CAD build for the part. Positions are in the model's coordinates, mm. Give positions to 0.01 mm unless a question says otherwise; leave off trailing zeros. Loops run counter-clockwise (first coordinate to the right, second up) from the corner with the lowest first, then second, coordinate; pieces in that order, holes last.
Item 1: Probe probe 1 along Z at (x, y) = (27, 2.75); probe 2 along X at (y, z) = (3.15, -56); probe 3 along Z at (x, y) = (-16, 2.35). List the from-to ranges inside material, lowest first.
Item 2: Saw through at C-C on x = -8. Give the cut face in (y, z).
Item 3: Drop flat-ended pins along their axis: P1, Ø5, axis at x = 25.54, z = -58.12, coming from the +Y side; P2, Ø2.5, axis at x = 25.54, z = 44.04, coming from the +Y side; P3, Ø2, axis at y = 1, z = -37.5, coming from the -X side. Give the stop position or say it passes through.
Item 4: Saw through at A-A on y = 3.2. Give the cut face in (x, z).
Item 5: Saw through at B-B on x = 63. Give the cut face in (y, z).
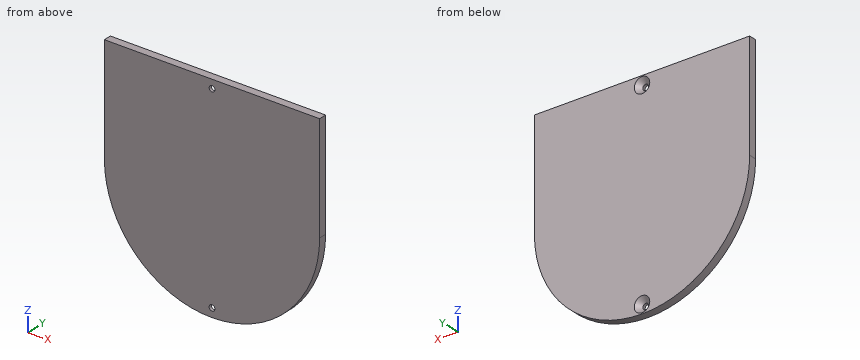
Autodesk Inventor part; units mm, degrees
ref_plane "YZ Plane" through (0, 0, 0) normal (1, 0, 0) x (0, 1, 0)
ref_plane "XZ Plane" through (0, 0, 0) normal (0, 1, 0) x (-1, 0, 0)
ref_plane "XY Plane" through (0, 0, 0) normal (0, 0, 1) x (1, 0, 0)
sketch "Sketch1" plane through (0, 0, 0) normal (0, 1, 0) x (-1, 0, 0)
  line L0 (30.0636, 48.5262) -> (-81.1364, 48.5262)
  line L1 (-81.1364, 48.5262) -> (-81.1364, -7.0738)
  line L2 (-81.1364, -7.0738) -> (30.0636, -7.0738)
  line L3 (30.0636, -7.0738) -> (30.0636, 48.5262)
  arc A0 (-81.1364, -7.0738) -> (30.0636, -7.0738) centre (-25.5364, -7.0738) ccw
  point P0 (0, 0)
  dimension "d0" = 55.6
  dimension "d1" = 111.2
  dimension "d2" = 55.6
extrude "Extrusion1" add sketch "Sketch1" along normal blind 4
sketch "Sketch2" plane through (0, 4, 0) normal (0, 1, 0) x (1, 0, 0)
  line L0 (-30.0636, 7.0738) -> (-30.0636, -48.5262)
  line L1 (-30.0636, -48.5262) -> (81.1364, -48.5262)
  point P0 (0, 0)
  point P1 (25.5364, -44.0432)
  dimension "d12" = 55.6
  dimension "d13" = 4.483
hole "Hole1" at (25.5364, 4, 44.0432) direction (0, -1, 0) diameter 3 depth 5 tip angle 118 countersink diameter 8 countersink angle 90
sketch "Sketch3" plane through (0, 4, 0) normal (0, 1, 0) x (1, 0, 0)
  line L0 (-30.0636, 7.0738) -> (-30.0636, -48.5262)
  arc A0 (81.1364, 7.0738) -> (-30.0636, 7.0738) centre (25.5364, 7.0738) ccw
  point P0 (0, 0)
  point P1 (25.5364, 58.1228)
  dimension "d21" = 55.6
  dimension "d22" = 51.049
hole "Hole2" at (25.5364, 4, -58.1228) direction (0, -1, 0) diameter 3 depth 5 tip angle 118 countersink diameter 8 countersink angle 90
properties part number "base-bottom-2"
Results below:
1. probe 1: z = -62.65 to -60.45, -55.79 to 41.72, 46.37 to 48.53
1. probe 2: x = -0.88 to 23.21, 27.86 to 51.95
1. probe 3: z = -44.03 to 48.53
2. outline: (0, -51.42) - (4, -51.42) - (4, 48.53) - (0, 48.53) - close
3. P1: stops at y = 2.5
3. P2: passes through
3. P3: stops at x = -21.64
4. outline: (-30.06, -7.07) arc R55.6 ccw to (81.14, -7.07) - (81.14, 48.53) - (-30.06, 48.53) - close; hole circle Ø6.4 at (25.54, -58.12); hole circle Ø6.4 at (25.54, 44.04)
5. outline: (0, -48.16) - (4, -48.16) - (4, 48.53) - (0, 48.53) - close
